Work out the finished part from the listing and answer in its coordinate system (mm). A direction names the side the tool comes from. Coordinates: 2 decimals unless noted, no trailing zeros. Order: outer loops, then holes, each group sorted by start corner. A loop starts at its lowest first (then second) coordinate and runs counter-clockwise, first axis right, second up. Notation, with made-up numbers: M 63,11 L 79,11 A20 ccw 79,44 Z; hole C 42,42.25 d5. An arc over 180 degrees is marked long. Use a Markdown table: item, result.
from build123d import *

# Parameters (mm, degrees)
SKETCH_1_R          = 3
EXTRUDE_1_DEPTH     = 4
SKETCH_6_R          = 0.5
EXTRUDE_2_DEPTH     = 2
SKETCH_3_R          = 2
CUT_EXTRUDE_2_DEPTH = 0.25
SKETCH_4_R          = 1.25
CUT_EXTRUDE_3_DEPTH = 4.75
SKETCH_2_R          = 2.5
CUT_EXTRUDE_1_DEPTH = 3.5


with BuildPart() as part:
    # 草图1 → 凸台-拉伸1 (new body)
    with BuildSketch(Plane.XY):
        Circle(SKETCH_1_R)
    extrude(amount=EXTRUDE_1_DEPTH)

    # 草图6 → 凸台-拉伸2 (add)
    with BuildSketch(Plane(origin=(0, 0, 0.25), x_dir=(-1, 0, 0), z_dir=(0, 0, -1))):
        with BuildLine():
            Line((-17, 2), (0, 3))
            Line((0, 3), (0, -3))
            Line((0, -3), (-17, -2))
            ThreePointArc((-17, -2), (-19, 0), (-17, 2))
        make_face()
        with Locations((-17.5, 0)):
            Circle(SKETCH_6_R, mode=Mode.SUBTRACT)
        with Locations((-15.5, 0)):
            Circle(SKETCH_6_R, mode=Mode.SUBTRACT)
        with Locations((-13.5, 0)):
            Circle(SKETCH_6_R, mode=Mode.SUBTRACT)
        with Locations((-11.5, 0)):
            Circle(SKETCH_6_R, mode=Mode.SUBTRACT)
        with Locations((-9.5, 0)):
            Circle(SKETCH_6_R, mode=Mode.SUBTRACT)
        with Locations((-7.5, 0)):
            Circle(SKETCH_6_R, mode=Mode.SUBTRACT)
        with Locations((-5.5, 0)):
            Circle(SKETCH_6_R, mode=Mode.SUBTRACT)
    extrude(amount=-EXTRUDE_2_DEPTH)

    # 草图3 → 切除-拉伸2 (cut)
    with BuildSketch(Plane(origin=(0, 0, 0), x_dir=(-1, 0, 0), z_dir=(0, 0, -1))):
        Circle(SKETCH_3_R)
    extrude(amount=-CUT_EXTRUDE_2_DEPTH, mode=Mode.SUBTRACT)

    # 草图4 → 切除-拉伸3 (cut, through all)
    with BuildSketch(Plane(origin=(0, 0, 0.25), x_dir=(-1, 0, 0), z_dir=(0, 0, -1))):
        Circle(SKETCH_4_R)
    extrude(amount=-CUT_EXTRUDE_3_DEPTH, mode=Mode.SUBTRACT)

    # 草图2 → 切除-拉伸1 (cut)
    with BuildSketch(Plane.XY.offset(4)):
        Circle(SKETCH_2_R)
    extrude(amount=-CUT_EXTRUDE_1_DEPTH, mode=Mode.SUBTRACT)


solid = part.part
1. Section C-C on y = -2.2 is taken. Determine the outline of the cut face in (x, z), then the cut area to 3 significant figures.
Answers below:
| item | result |
|---|---|
| outline | M -2.04,0 L 2.04,0 L 2.04,0.25 L 13.6,0.25 L 13.6,2.25 L 2.04,2.25 L 2.04,4 L 1.19,4 L 1.19,0.5 L -1.19,0.5 L -1.19,4 L -2.04,4 Z |
| area | 31.1 mm² |
2. Section B-B on z = 2.9 is taken. Determine the outline of the cut face in (x, y), then the cut area to 3 significant figures.
Answers below:
| item | result |
|---|---|
| outline | C 0,0 d6; hole C 0,0 d5 |
| area | 8.64 mm² |
3. Find the intervals of material crossed by probe 1 along Y at (x, z) = (0, 3.15); probe 2 along Y at (x, z) = (0, 0.45); probe 3 along Z at (x, y) = (6, 0.35), in increasing order.
Answers below:
| item | result |
|---|---|
| probe 1 | -3 to -2.5, 2.5 to 3 |
| probe 2 | -3 to -1.25, 1.25 to 3 |
| probe 3 | 0.25 to 2.25 |
4. For a pull along X with two mould halves and no side action, classify faces 3 (the face through (-2, 2, 4)), 4 (the face through (-1, 1, 0.25)), 5 (the face through (8.792, 2.483, 1.236)) as +X half, -X half, draft (parallel to the pull), parting line (faces both ways), or undercut.
Answers below:
| item | result |
|---|---|
| face 3 | draft |
| face 4 | undercut |
| face 5 | +X half |
5. Section D-D on x = 7.5 is taken. Determine the outline of the cut face in (y, z), then the cut area to 3 significant figures.
Answers below:
| item | result |
|---|---|
| outline | M -2.56,0.25 L -0.5,0.25 L -0.5,2.25 L -2.56,2.25 Z; M 0.5,0.25 L 2.56,0.25 L 2.56,2.25 L 0.5,2.25 Z |
| area | 8.24 mm² |
6. Section A-A on x = 0 is taken. Determine the outline of the cut face in (y, z), then the cut area to 4 significant figures.
Answers below:
| item | result |
|---|---|
| outline | M -3,0 L -2,0 L -2,0.25 L -1.25,0.25 L -1.25,0.5 L -2.5,0.5 L -2.5,4 L -3,4 Z; M 1.25,0.25 L 2,0.25 L 2,0 L 3,0 L 3,4 L 2.5,4 L 2.5,0.5 L 1.25,0.5 Z |
| area | 4.875 mm² |
7. For faces 1 (the face through (-1, -1, 0.5)), 2 (the face through (12, 0, 1)), determine the directions among +Z, -Z, +X, -X, +Y, -Y from which every point of the face is accessible in a straight line to the end or side of a thin tool.
Answers below:
| item | result |
|---|---|
| face 1 | +Z |
| face 2 | +Z, -Z |
8. Flat-ended cylindrical pins translate along their axes: P1, Ø3, axis at x = 16.5, y = 1.5, coming from the +Z side; P2, Ø3, axis at x = 0, y = 0, coming from the -Z side; P3, Ø2, axis at y = 1.5, z = 1.5, coming from the -X side. Find the tip coordinate at first contact, or state that the pin passes through.
Answers below:
| item | result |
|---|---|
| P1 | z = 2.25 |
| P2 | z = 0.25 |
| P3 | x = -2.96 |
